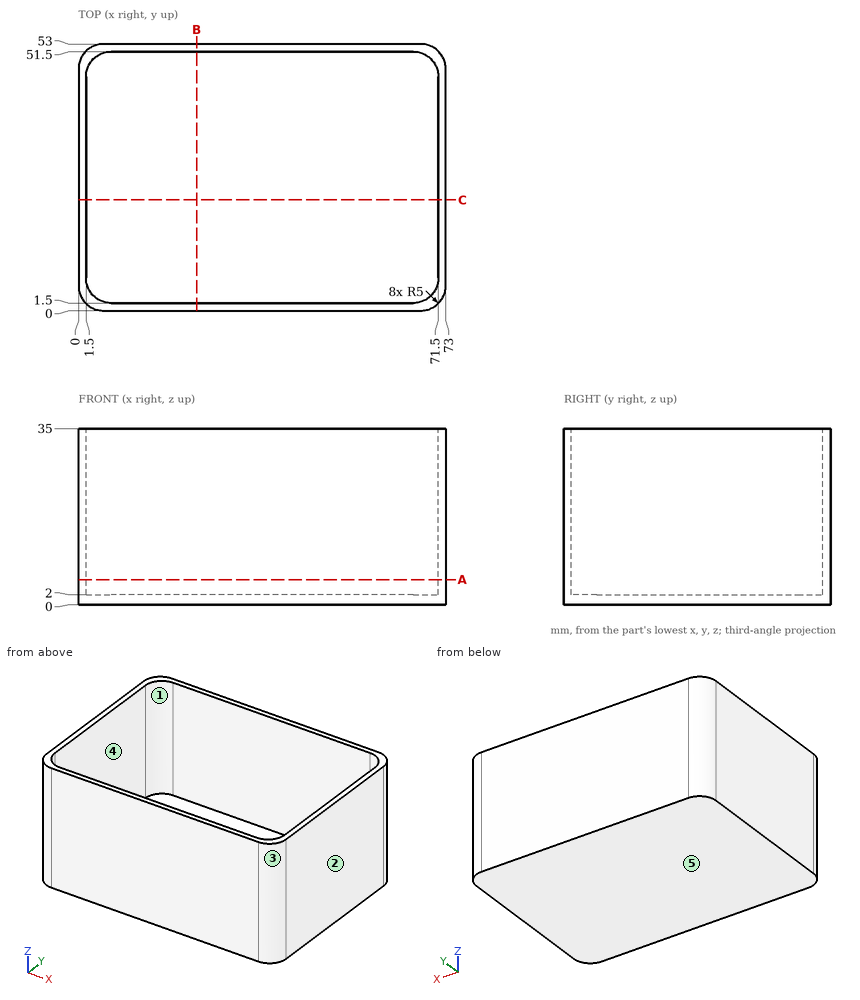
Job drawing, mm, ordinate dimensions from the low corner. One solid piece. A direction names the side the tool comes from. Round coordinates to 2 decimals unless told otherwise and drop trailing zeros. Write each loop counter-clockwise with the first axis right and the second up, starting at its lowest first coordinate (ties: lowest second). Pieces come first, ordered by that corner, then holes.
1) Mould opens along Y. For the marked faces 1, 2 and 3 say: +Y half, -Y half, draft (parallel to the pull), parting line (faces both ways), or undercut.
2) 3-axis set-ups, long thin cutter, end or side, ignore diameter. For the marked faces 4 and 5: which of +Z, -Z, +X, -X, +Y, -Y reach the whole face in a straight line?
3) Drill centre lines: probe 1 along X at (y, z) = (18, 22); probe 2 along Y at (x, z) = (60.5, 12); probe 3 along Z at (x, y) = (12, 10.5). Where is each one in solid material? Low to high.
4) Band-saw the part on C-C, the plane y = 22. List the corners of the cut face in (x, z), and give its area (3 significant figures).
5) Pin check, flat tips, straight feed: pin 1 (15 mm diameter, centred on x = 31.5, y = 37, fed in from +Z); pin 2 (4 mm diameter, centred on y = 22.5, z = 13, fed in from -X). Stop position of each tip, or through.
6) Band-saw the part on A-A, the plane z = 5. List the corners of the cut face in (x, y).
7) Band-saw the part on B-B, the plane x = 23.5. List the corners of the cut face in (y, z), and give its area (3 significant figures).
Ans:
1. face 1: undercut
1. face 2: draft
1. face 3: -Y half
2. face 4: +Z
2. face 5: -Z, +X, -X, +Y, -Y
3. probe 1: x = 0 to 1.5, 71.5 to 73
3. probe 2: y = 0 to 1.5, 51.5 to 53
3. probe 3: z = 0 to 2
4. outline: (0, 0) - (73, 0) - (73, 35) - (71.5, 35) - (71.5, 2) - (1.5, 2) - (1.5, 35) - (0, 35) - close
4. area: 245 mm2
5. pin 1: stops at z = 2
5. pin 2: stops at x = 0
6. outline: (0, 5) arc R5 ccw to (5, 0) - (68, 0) arc R5 ccw to (73, 5) - (73, 48) arc R5 ccw to (68, 53) - (5, 53) arc R5 ccw to (0, 48) - close; hole (1.5, 6.5) arc R5 ccw to (6.5, 1.5) - (66.5, 1.5) arc R5 ccw to (71.5, 6.5) - (71.5, 46.5) arc R5 ccw to (66.5, 51.5) - (6.5, 51.5) arc R5 ccw to (1.5, 46.5) - close
7. outline: (0, 0) - (53, 0) - (53, 35) - (51.5, 35) - (51.5, 2) - (1.5, 2) - (1.5, 35) - (0, 35) - close
7. area: 205 mm2
